from build123d import *

# Parameters (mm, degrees)
SKETCH1_W           = 40
SKETCH1_H           = 250
SKETCH1_R           = 4
BOSS_EXTRUDE1_DEPTH = 4
CHAMFER1_SIZE       = 3.5
CHAMFER3_SIZE       = 20


with BuildPart() as part:
    # Sketch1 → Boss-Extrude1 (new body)
    with BuildSketch(Plane(origin=(0, 0, 0), x_dir=(0, 0, -1), z_dir=(1, 0, 0))):
        Rectangle(SKETCH1_W, SKETCH1_H)
        with Locations((0, 105)):
            Circle(SKETCH1_R, mode=Mode.SUBTRACT)
        with Locations((0, -105)):
            Circle(SKETCH1_R, mode=Mode.SUBTRACT)
    extrude(amount=BOSS_EXTRUDE1_DEPTH)

    # Chamfer1
    chamfer1_edges = [part.edges().sort_by_distance(p)[0] for p in [
        (0, 105, 4),
    ]]
    chamfer(chamfer1_edges, length=CHAMFER1_SIZE)

    # Chamfer3
    chamfer3_edges = [part.edges().sort_by_distance(p)[0] for p in [
        (2, -125, -20),
    ]]
    chamfer(chamfer3_edges, length=CHAMFER3_SIZE)


solid = part.part
Input: part model. Units: mm. Frame: model coordinates. Give positions to 0.01 mm unless a question says otherwise; leave off trailing zeros. Loops run counter-clockwise (first coordinate to the right, second up) from the corner with the lowest first, then second, coordinate; pieces in that order, holes last. Notation, with made-up numbers: (-36, -35.5) -> (19, -35.5) arc R18 ccw to (19, -5.5) -> close; hole circle Ø4 at (28.25, 85.5). An arc over 180 degrees is marked (long way). Answer as a JSON object with one key per item and string values. Group by question number.
Item 1: Pull-direction query (Z, two-part tool) for faces 1 (the flat face through (2, 8, -20)), 2 (the conical face through (3.281, 109.183, 0.549)), 3 (the flat face through (2, 125, 0)), 4 (the cylindrical face through (3.746, 101.451, -1.846)); classes: released by +Z, released by -Z, zero draft, split by the parting line, or undercut.
Item 2: Line query: probe 1 along Y at (x, z) = (0.85, -6); probe 2 along Y at (x, z) = (1, 5); probe 3 along Z at (x, y) = (2.8, -101.5). Output: solid intervals per line, ascending.
Item 3: Cut plane A-A, the plane y = 105. Return the cut outline in (x, z).
Item 4: Cut plane B-B, the plane x = 0.7. Return the cut outline in (y, z), and give its area (3 significant figures).
Item 5: Pin query (flat end, axial travel): P1, Ø5, axis at y = 105, z = 0, coming from the -X side; P2, Ø2, axis at y = -66.5, z = -2.5, coming from the -X side; P3, Ø1.5, axis at x = 2.5, z = -5.5, coming from the -Y side. Return the tip coordinate at first contact, or that it passes through.
Item 6: Cut plane C-C, the plane z = -13. Return the cut outline in (x, y), and give its area (3 significant figures).
Checks:
{
 "1": {"face 1": "released by -Z", "face 2": "undercut", "face 3": "zero draft", "face 4": "undercut"},
 "2": {"probe 1": "y = -119 to 102.13, 107.87 to 125", "probe 2": "y = -125 to 100.85, 109.15 to 125", "probe 3": "z = -20 to -1.94, 1.94 to 20"},
 "3": {"outline": "(0, -20) -> (4, -20) -> (4, -4) -> (3.5, -4) -> (0, -7.5) -> close; (0, 7.5) -> (3.5, 4) -> (4, 4) -> (4, 20) -> (0, 20) -> close"},
 "4": {"outline": "(-125, 0) -> (-105, -20) -> (125, -20) -> (125, 20) -> (-125, 20) -> close; hole circle Ø8 at (-105, 0); hole circle Ø13.6 at (105, 0)", "area": "9,600 mm²"},
 "5": {"P1": "passes through", "P2": "stops at x = 0", "P3": "stops at y = -120.25"},
 "6": {"outline": "(0, -112) -> (4, -112) -> (4, 125) -> (0, 125) -> close", "area": "948 mm²"}
}
